```python
from build123d import *

# Parameters (mm, degrees)
SKETCH1_R           = 1.51
BOSS_EXTRUDE1_DEPTH = 47
SKETCH4_R           = 2.475
BOSS_EXTRUDE2_DEPTH = 10
FILLET1_R           = 0.3


with BuildPart() as part:
    # Sketch1 → Boss-Extrude1 (new body)
    with BuildSketch(Plane(origin=(0, 0, 0), x_dir=(1, 0, 0), z_dir=(0, 1, 0))):
        Polygon((-17.01, 21.15), (-21.15, 17.01), (-21.15, -17.01), (-17.01, -21.15), (17.01, -21.15), (21.15, -17.01), (21.15, 17.01), (17.01, 21.15), align=None)
        with Locations(Location((15.5, 15.5, 0), (0, 0, 270))):
            Circle(SKETCH1_R, mode=Mode.SUBTRACT)
        with Locations(Location((15.5, -15.5, 0), (0, 0, 270))):
            Circle(SKETCH1_R, mode=Mode.SUBTRACT)
        with Locations(Location((-15.5, -15.5, 0), (0, 0, 270))):
            Circle(SKETCH1_R, mode=Mode.SUBTRACT)
        with Locations(Location((-15.5, 15.5, 0), (0, 0, 270))):
            Circle(SKETCH1_R, mode=Mode.SUBTRACT)
    extrude(amount=BOSS_EXTRUDE1_DEPTH)

    # Sketch4 → Boss-Extrude2 (add)
    with BuildSketch(Plane(origin=(0, 0, 0), x_dir=(1, 0, 0), z_dir=(0, 1, 0))):
        with Locations(Location((0, 0, 0), (0, 0, 270))):
            Circle(SKETCH4_R)
    extrude(amount=-BOSS_EXTRUDE2_DEPTH)

    # Fillet1
    fillet1_edges = [part.edges().sort_by_distance(p)[0] for p in [
        (0, -10, -2.475),
    ]]
    fillet(fillet1_edges, radius=FILLET1_R)


solid = part.part
```
Geometry: final body of the model. Coordinates: model frame, mm. A direction names the side the tool comes from. Round coordinates to 2 decimals unless told otherwise and drop trailing zeros. Order: outer loops, then holes, each group sorted by start corner. A loop starts at its lowest first (then second) coordinate and runs counter-clockwise, first axis right, second up. Notation, with made-up numbers: (13.25, 16) -> (34.25, 16) arc R13 ccw to (34.25, 40) -> close; hole circle Ø5 at (12.25, 19.5). An arc over 180 degrees is marked (long way). Use CSV: the item, a comma, the result in double quotes. Start each with the question number.
1) Section B-B (x = -15.5). Return the cut outline in (y, z).
2) Section C-C (y = 11). Return the cut outline in (x, z).
3) Material intervals for line 1 along X through (y, z) = (31.5, 15.5); line 2 along Z through (x, y) = (-15, 24); line 3 along Y through (x, z) = (3.5, 6), sorted ascending. Write a range as from..to.
4) Section A-A (z = -15.5). Return the cut outline in (x, y), and give its area (3 significant figures).
5) Section D-D (z = 0). Return the cut outline in (x, y) (3 decimals).
6) First-contact query: pin 1 Ø4 at (x, z) = (15.5, 15.5) entering from -Y. Flat tip, straight axial feed; report the tip coordinate or a pass-through.
7) Draft query along X for faces 1 (the face through (21.15, 23, 0)), 2 (the face through (0, 23, -21.15)), 3 (the face through (14.026, 23.171, 15.173)), 4 (the face through (-16.974, 23.171, -15.827)). Return one class per face: +X half, -X half, draft (parallel to the pull), parting line (faces both ways), or undercut.
8) Set-up query: faces 5 (the face through (0, -10, 0)), 6 (the face through (0.74, -4.78, 2.36)). Return all of +Z, -Z, +X, -X, +Y, -Y with unobstructed straight access to the full face (end or side cutting, diameter ignored); none if empty.
Returned:
1,outline,"(0, -21.15) -> (47, -21.15) -> (47, -17.01) -> (0, -17.01) -> close; (0, -13.99) -> (47, -13.99) -> (47, 13.99) -> (0, 13.99) -> close; (0, 17.01) -> (47, 17.01) -> (47, 21.15) -> (0, 21.15) -> close"
2,outline,"(-21.15, -17.01) -> (-17.01, -21.15) -> (17.01, -21.15) -> (21.15, -17.01) -> (21.15, 17.01) -> (17.01, 21.15) -> (-17.01, 21.15) -> (-21.15, 17.01) -> close; hole circle Ø3.02 at (-15.5, -15.5); hole circle Ø3.02 at (-15.5, 15.5); hole circle Ø3.02 at (15.5, -15.5); hole circle Ø3.02 at (15.5, 15.5)"
3,line 1,"x = -21.15..-17.01, -13.99..13.99, 17.01..21.15"
3,line 2,"z = -21.15..-16.92, -14.08..14.08, 16.92..21.15"
3,line 3,"y = 0..47"
4,outline,"(-21.15, 0) -> (-17.01, 0) -> (-17.01, 47) -> (-21.15, 47) -> close; (-13.99, 0) -> (13.99, 0) -> (13.99, 47) -> (-13.99, 47) -> close; (17.01, 0) -> (21.15, 0) -> (21.15, 47) -> (17.01, 47) -> close"
4,area,"1,700 mm²"
5,outline,"(-21.15, 0) -> (-2.475, 0) -> (-2.475, -9.7) arc R0.3 ccw to (-2.175, -10) -> (2.175, -10) arc R0.3 ccw to (2.475, -9.7) -> (2.475, 0) -> (21.15, 0) -> (21.15, 47) -> (-21.15, 47) -> close"
6,pin 1,"stops at y = 0"
7,face 1,"+X half"
7,face 2,"draft"
7,face 3,"undercut"
7,face 4,"undercut"
8,face 5,"+Z, -Z, +X, -X, -Y"
8,face 6,"-Y"
